Source: CAD feature listing. Evaluate the final solid. Frame: model axes, mm. Face numbers are marked on the shaded views. A direction names the side the tool comes from. Coordinates: 2 decimals unless noted, no trailing zeros. Write each loop counter-clockwise with the first axis right and the second up, starting at its lowest first coordinate (ties: lowest second). Pieces come first, ordered by that corner, then holes. Notation, with made-up numbers: M -4,57.5 L 24,57.5 A8 ccw 24,66.5 Z; hole C 29,74 d8. An arc over 180 degrees is marked long. Write item = value, one per line. Start each with the question number.
1. Section query D-D (y = -168). Output: boundary loops of the cut face in (x, z).
2. Section query A-A (x = 197.5). Output: boundary loops of the cut face in (y, z), then the cut area to 3 significant figures.
3. Pin query (flat end, axial travel): pin 1 Ø4 at (x, z) = (31.5, 150) entering from +Y; pin 2 Ø5 at (x, z) = (163.5, 176.5) entering from -Y; pin 3 Ø1 at (y, z) = (-129.5, 131.5) entering from -X. Return the tip coordinate at first contact, or that it passes through.
4. Access query for the marked faces 1 and 2. Directions: +Z, -Z, +X, -X, +Y, -Y. A direction counts if a zero-diameter tool reaches every point of the face in a straight line with its end or side. Return the directions, or none.
5. Section query B-B (z = 88). Output: boundary loops of the cut face in (x, y), then the cut area to 3 significant figures.
6. Line query: line 1 along X through (y, z) = (-111, 46.5); line 2 along Y through (x, z) = (204, 33); line 3 along Y through (x, z) = (159.5, 176). Output: solid intervals per line, ascending.
7. Section query C-C (x = 32). Output: boundary loops of the cut face in (y, z), then the cut area to 3 significant figures.
```python
from build123d import *

# Parameters (mm, degrees)
SKETCH1_W           = 25
SKETCH1_H           = 120
BOSS_EXTRUDE4_DEPTH = 200


with BuildPart() as part:
    # Sketch1 → Boss-Extrude4 (new body)
    with BuildSketch(Plane.XY):
        with Locations((-12.5, -60)):
            Rectangle(SKETCH1_W, SKETCH1_H)
        Polygon((-25, -120), (0, -120), (191.51111078, -280.696902422), (166.51111078, -280.696902422), align=None)
        Polygon((233.990264512, -245.068874008), (149.051279921, -245.068874008), (157.072044946, -251.799094983), (233.990264512, -251.799094983), align=None)
        Polygon((191.51111078, -280.696902422), (235.34462255, -280.696902422), (235.34462255, -274.614068302), (184.261871365, -274.614068302), align=None)
    extrude(amount=BOSS_EXTRUDE4_DEPTH)


solid = part.part
```
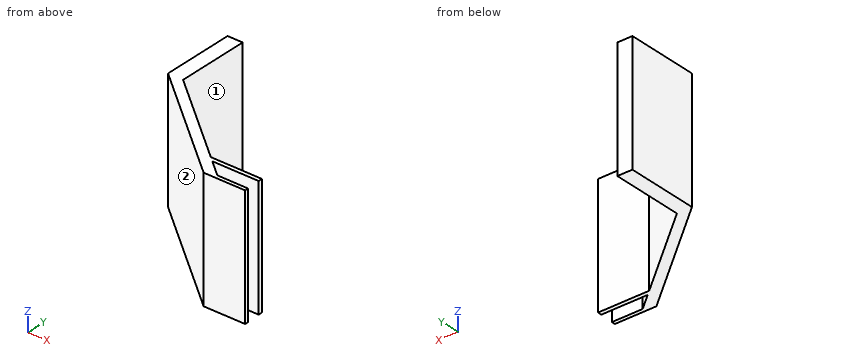
Results are:
q1.outline = M 32.2,0 L 57.2,0 L 57.2,200 L 32.2,200 Z
q2.outline = M -280.7,0 L -274.61,0 L -274.61,200 L -280.7,200 Z; M -251.8,0 L -245.07,0 L -245.07,200 L -251.8,200 Z
q2.area = 2,560 mm^2
q3.pin_1 = -144.75
q3.pin_2 = -280.27
q3.pin_3 = -14.27
q4.face_1 = +Z, -Z, +X, +Y
q4.face_2 = +Z, -Z, -X, -Y
q5.outline = M -25,-120 L 166.51,-280.7 L 235.34,-280.7 L 235.34,-274.61 L 184.26,-274.61 L 157.07,-251.8 L 233.99,-251.8 L 233.99,-245.07 L 149.05,-245.07 L 0,-120 L 0,0 L -25,0 Z
q5.area = 7,850 mm^2
q6.line_1 = -25 to 0
q6.line_2 = -280.7 to -274.61, -251.8 to -245.07
q6.line_3 = -274.81 to -253.84, -251.8 to -245.07
q7.outline = M -167.83,0 L -146.85,0 L -146.85,200 L -167.83,200 Z
q7.area = 4,200 mm^2
